Autodesk Inventor part; units mm, degrees
ref_plane "YZ Plane" through (0, 0, 0) normal (1, 0, 0) x (0, 1, 0)
ref_plane "XZ Plane" through (0, 0, 0) normal (0, 1, 0) x (-1, 0, 0)
ref_plane "XY Plane" through (0, 0, 0) normal (0, 0, 1) x (1, 0, 0)
sketch "Sketch1" plane through (0, 0, 0) normal (0, 0, 1) x (1, 0, 0)
  line L0 (0, 0) -> (100, 0)
  line L1 (100, 0) -> (100, 150)
  line L2 (100, 150) -> (0, 150)
  line L3 (0, 150) -> (0, 0)
  circle A0 centre (50, 207.5) radius 37.5
  line L4 (-20, -20) -> (120, -20)
  line L5 (120, -20) -> (120, 170)
  line L6 (120, 170) -> (-20, 170)
  line L7 (-20, 170) -> (-20, -20)
  line L8 (0, 170) -> (100, 170)
  line L9 (49.5, -20) -> (59.5, -20)
  line L10 (45, -20) -> (60, -20)
  line L11 (42.5, -20) -> (57.5, -20)
  line L12 (57.5, -20) -> (57.5, -35)
  line L13 (57.5, -35) -> (42.5, -35)
  line L14 (42.5, -35) -> (42.5, -20)
  line L15 (100, 170) -> (100, 207.5)
  line L16 (100, 207.5) -> (87.5, 207.5)
  line L17 (0, 170) -> (0, 207.5)
  line L18 (0, 207.5) -> (12.5, 207.5)
  dimension "d0" = 75
  dimension "d1" = 140
  dimension "d3" = 15
  dimension "d4" = 15
extrude "Extrusion1" add sketch "Sketch1" along normal blind 5.5 contours L16 L15 L6 A0 | A0 L6 L17 L18 | L6 L5 L4 L7 | L4 L12 L13 L14
properties part number "anillo4"
Model file for the job. Use its own axes, mm. A direction names the side the tool comes from. Coordinates: 2 decimals unless noted, no trailing zeros. Order: outer loops, then holes, each group sorted by start corner. A loop starts at its lowest first (then second) coordinate and runs counter-clockwise, first axis right, second up. Notation, with made-up numbers: (34.25, 22.5) - (86.25, 22.5) arc R15 ccw to (86.25, 43.5) - close; hole circle Ø9 at (75, 77.25). An arc over 180 degrees is marked (long way). Return JSON: item names as keys, results as strings. Group by question number.
1) Saw through at A-A, the plane y = 141.5. Write the cut outline in (x, z), plus the area to 3 significant figures.
2) Flat gauge pins, fed straight in: P1, Ø2, axis at x = 73, z = 3, coming from the +Y side; P2, Ø3, axis at x = 83.5, z = 2.5, coming from the -Y side; P3, Ø10, axis at x = 21.5, y = -5.5, coming from the -Z side; P4, Ø3, axis at x = 31, z = 2.5, coming from the +Y side. Where does each tip first touch, or does it go through?
3) Probe line 1 (X direction, y = 32, z = 1.3); line 2 (Y direction, x = 99.5, z = 4.9); line 3 (Y direction, x = 50, z = 3.15). List the from-to ranges inside material, lowest first. Write a range as from..to.
4) Saw through at D-D, the plane x = -9.5. Write the cut outline in (y, z), plus the area to 4 significant figures.
5) Saw through at C-C, the plane x = 50. Write the cut outline in (y, z).
6) Saw through at B-B, the plane z = 1.3. Write the cut outline in (x, y).
7) Tool access for faces 4 (the flat face through (57.5, -27, 3)), 5 (the flat face through (0, 188, 3)), 6 (the flat face through (49, 0, 3)), 7 (the flat face through (42.5, -28, 3)), 8 (the flat face through (110, 170, 3)): list every direction of +Z, -Z, +X, -X, +Y, -Y with a clear straight run to the whole face (end or side of a thin tool).
8) Mould opens along X. For faces 1 (the flat face through (88, -20, 3)), 2 (the flat face through (120, 74, 3)), 3 (the flat face through (100, 74, 3)) say: released by +X, released by -X, zero draft, split by the parting line, or undercut.
Values found:
{
 "1": {"outline": "(-20, 0) - (0, 0) - (0, 5.5) - (-20, 5.5) - close; (100, 0) - (120, 0) - (120, 5.5) - (100, 5.5) - close", "area": "220 mm²"},
 "2": {"P1": "stops at y = 178.69", "P2": "stops at y = -20", "P3": "stops at z = 0", "P4": "stops at y = 176.1"},
 "3": {"line 1": "x = -20..0, 100..120", "line 2": "y = -20..0, 150..207.5", "line 3": "y = -35..0, 150..170"},
 "4": {"outline": "(-20, 0) - (170, 0) - (170, 5.5) - (-20, 5.5) - close", "area": "1,045 mm²"},
 "5": {"outline": "(-35, 0) - (0, 0) - (0, 5.5) - (-35, 5.5) - close; (150, 0) - (170, 0) - (170, 5.5) - (150, 5.5) - close"},
 "6": {"outline": "(-20, -20) - (42.5, -20) - (42.5, -35) - (57.5, -35) - (57.5, -20) - (120, -20) - (120, 170) - (100, 170) - (100, 207.5) - (87.5, 207.5) arc R37.5 cw to (12.5, 207.5) - (0, 207.5) - (0, 170) - (-20, 170) - close; hole (0, 0) - (100, 0) - (100, 150) - (0, 150) - close"},
 "7": {"face 4": "+Z, -Z, +X, -Y", "face 5": "+Z, -Z, -X, +Y", "face 6": "+Z, -Z", "face 7": "+Z, -Z, -X, -Y", "face 8": "+Z, -Z, +X, +Y"},
 "8": {"face 1": "zero draft", "face 2": "released by +X", "face 3": "undercut"}
}
